Job drawing, mm, ordinate dimensions from the low corner. One solid piece. Round coordinates to 2 decimals unless told otherwise and drop trailing zeros. Order: outer loops, then holes, each group sorted by start corner. A loop starts at its lowest first (then second) coordinate and runs counter-clockwise, first axis right, second up. Notation, with made-up numbers: (86, 48) -> (99, 48) arc R14 cw to (99, 67) -> close; hole circle Ø5 at (-27, 20). An arc over 180 degrees is marked (long way). Answer as a JSON object with one key per item and string values. Group by question number.
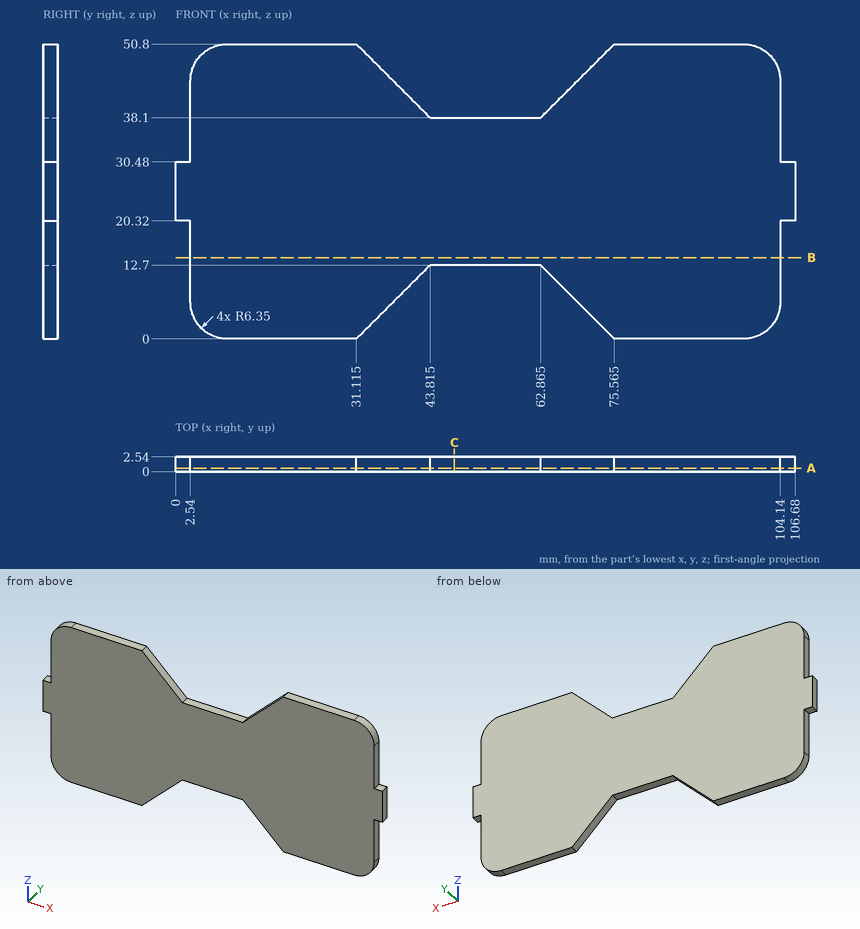
Q1. Wall check: line 1 (Z direction, x = 44, y = 2); line 2 (X direction, y = 1.85, z = 37.5); line 3 (X direction, y = 1.9, z = 40) (3 decimals). Give the ranges that are in metal, low to high. Write a range as [from, to].
Q2. Band-saw the part on C-C (x = 48). List the corners of the cut face in (y, z).
Q3. Band-saw the part on B-B (z = 14). List the corners of the cut face in (x, y), plus the area to 3 significant figures.
Q4. Drop flat-ended pins along their axis: pin 1 Ø1.3 at (x, y) = (106, 1) entering from -Z; pin 2 Ø1.3 at (y, z) = (2, 37.5) entering from +X; pin 3 Ø1.5 at (y, z) = (1, 44) entering from -X. Give the stop position or say it passes through.
Q5. Band-saw the part on A-A (y = 0.6). List the corners of the cut face in (x, z) (3 decimals), plus the area to 3 significant figures.
Completed:
{
 "1": {"line 1": "[12.7, 38.1]", "line 2": "[2.54, 104.14]", "line 3": "[2.54, 41.915], [64.765, 104.14]"},
 "2": {"outline": "(0, 12.7) -> (2.54, 12.7) -> (2.54, 38.1) -> (0, 38.1) -> close"},
 "3": {"outline": "(2.54, 0) -> (104.14, 0) -> (104.14, 2.54) -> (2.54, 2.54) -> close", "area": "258 mm2"},
 "4": {"pin 1": "z = 20.32", "pin 2": "x = 104.14", "pin 3": "x = 2.54"},
 "5": {"outline": "(0, 20.32) -> (2.54, 20.32) -> (2.54, 6.35) arc R6.35 ccw to (8.89, 0) -> (31.115, 0) -> (43.815, 12.7) -> (62.865, 12.7) -> (75.565, 0) -> (97.79, 0) arc R6.35 ccw to (104.14, 6.35) -> (104.14, 20.32) -> (106.68, 20.32) -> (106.68, 30.48) -> (104.14, 30.48) -> (104.14, 44.45) arc R6.35 ccw to (97.79, 50.8) -> (75.565, 50.8) -> (62.865, 38.1) -> (43.815, 38.1) -> (31.115, 50.8) -> (8.89, 50.8) arc R6.35 ccw to (2.54, 44.45) -> (2.54, 30.48) -> (0, 30.48) -> close", "area": "4,370 mm2"}
}
